```python
from build123d import *

# Parameters (mm, degrees)
ESBO_O1_R                  = 1.75
ESBO_O1_R_2                = 11.5
ESBO_O1_R_3                = 4
ESBO_O1_R_4                = 2.25
RESSALTO_EXTRUS_O1_DEPTH   = 30
ESBO_O2_W                  = 43
ESBO_O2_H                  = 43
ESBO_O2_W_2                = 5.1
ESBO_O2_H_2                = 3
CORTE_EXTRUS_O1_DEPTH      = 22
ESBO_O3_R                  = 4.5
CORTE_EXTRUS_O2_DEPTH      = 3
CORTE_EXTRUS_O3_DEPTH      = 68.950349521
CORTE_EXTRUS_O3_DEPTH_BACK = 3
ESBO_O4_R                  = 1.5


with BuildPart() as part:
    # Esboço1 → Ressalto-extrusão1 (new body)
    with BuildSketch(Plane.XY):
        with BuildLine():
            Line((-26, 26), (26, 26))
            Line((26, 26), (47.462602, 10.027939539))
            ThreePointArc((47.462602, 10.027939539), (52.5, 0), (47.462602, -10.027939539))
            Line((47.462602, -10.027939539), (26, -26))
            Line((26, -26), (-26, -26))
            Line((-26, -26), (-47.462602, -10.027939539))
            ThreePointArc((-47.462602, -10.027939539), (-52.5, 0), (-47.462602, 10.027939539))
            Line((-47.462602, 10.027939539), (-26, 26))
        make_face()
        with Locations((-15.5, 15.5)):
            Circle(ESBO_O1_R, mode=Mode.SUBTRACT)
        with Locations((15.5, 15.5)):
            Circle(ESBO_O1_R, mode=Mode.SUBTRACT)
        with Locations((15.5, -15.5)):
            Circle(ESBO_O1_R, mode=Mode.SUBTRACT)
        with Locations((-15.5, -15.5)):
            Circle(ESBO_O1_R, mode=Mode.SUBTRACT)
        Circle(ESBO_O1_R_2, mode=Mode.SUBTRACT)
        with Locations((-40, 0)):
            Circle(ESBO_O1_R_3, mode=Mode.SUBTRACT)
        with Locations((40, 0)):
            Circle(ESBO_O1_R_3, mode=Mode.SUBTRACT)
        with Locations((-32.5, 7.5)):
            Circle(ESBO_O1_R_4, mode=Mode.SUBTRACT)
        with Locations((-32.5, -7.5)):
            Circle(ESBO_O1_R_4, mode=Mode.SUBTRACT)
        with Locations(Location((32.5, -7.5, 0), (0, 0, 180))):
            Circle(ESBO_O1_R_4, mode=Mode.SUBTRACT)
        with Locations(Location((32.5, 7.5, 0), (0, 0, 180))):
            Circle(ESBO_O1_R_4, mode=Mode.SUBTRACT)
    extrude(amount=RESSALTO_EXTRUS_O1_DEPTH)

    # Esboço2 → Corte-extrusão1 (cut)
    with BuildSketch(Plane.XY.offset(30)):
        Rectangle(ESBO_O2_W, ESBO_O2_H)
        with Locations((-40, 6.5)):
            Rectangle(ESBO_O2_W_2, ESBO_O2_H_2)
        with Locations((40, 6.5)):
            Rectangle(ESBO_O2_W_2, ESBO_O2_H_2)
    extrude(amount=-CORTE_EXTRUS_O1_DEPTH, mode=Mode.SUBTRACT)

    # Esboço3 → Corte-extrusão2 (cut)
    with BuildSketch(Plane(origin=(0, 0, 0), x_dir=(-1, 0, 0), z_dir=(0, 0, -1))):
        with Locations((-15.5, 15.5)):
            Circle(ESBO_O3_R)
        with Locations((15.5, 15.5)):
            Circle(ESBO_O3_R)
        with Locations((-15.5, -15.5)):
            Circle(ESBO_O3_R)
        with Locations((15.5, -15.5)):
            Circle(ESBO_O3_R)
    extrude(amount=-CORTE_EXTRUS_O2_DEPTH, mode=Mode.SUBTRACT)

    # Esboço4 → Corte-extrusão3 (cut, two sides: drawn at the far end of the back side and taken through both)
    with BuildSketch(Plane(origin=(0, 5, 0), x_dir=(1, 0, 0), z_dir=(0, 1, 0)).offset(-CORTE_EXTRUS_O3_DEPTH_BACK)):
        with Locations(Location((-40, -19, 0), (0, 0, 180))):
            Circle(ESBO_O4_R)
        with Locations((40, -19)):
            Circle(ESBO_O4_R)
    extrude(amount=CORTE_EXTRUS_O3_DEPTH + CORTE_EXTRUS_O3_DEPTH_BACK, mode=Mode.SUBTRACT)


solid = part.part
```
Source: CAD feature listing. Evaluate the final solid. Frame: model axes, mm. A direction names the side the tool comes from. Coordinates: 2 decimals unless noted, no trailing zeros. Loops run counter-clockwise (first coordinate to the right, second up) from the corner with the lowest first, then second, coordinate; pieces in that order, holes last. Notation, with made-up numbers: M 21.5,-30 L 56.5,-30 A14 cw 56.5,-11 Z; hole C 39,34.25 d7. An arc over 180 degrees is marked long. Use a Markdown table: item, result. Add a question column.
Q1. Draft query along X for faces 5 (the flat face through (36.882, -17.902, 14.79)), 6 (the cylindrical face through (30.354, 6.824, 14.79)), 7 (the flat face through (-36.581, -18.126, 14.79)). Return one class per face: pulls with the +X half, pulls with the -X half, needs draft (parallel to the pull), parting line crosses it, or undercut.
Q2. Section query C-C, the plane x = 15.5. Return loops of the section in (y, z).
Q3. Section query A-A, the plane x = 0. Return loops of the section in (y, z).
Q4. Material intervals for L1, parallel to Y at x = -15.5, z = 1.65; L2, parallel to Y at x = 0, z = 5; L3, parallel to Y at x = -2, z = 17, sorted ascending.
Q5. Access query for faces 1 (the flat face through (-37.45, 6, 19)), 2 (the cylindrical face through (-41.43, 4.49, 19.45)), 3 (the flat face through (-17.4, -15.4, 3)), 4 (the cylindrical face through (-14.6, -14, 5.5)). Directions: +Z, -Z, +X, -X, +Y, -Y. A direction counts if a zero-diameter tool reaches every point of the face in a straight line with its end or side. Return the directions, or none.
Q6. First-contact query: pin 1 (2.5 mm diameter, centred on x = -40, y = 7, fed in from +Z); pin 2 (2.5 mm diameter, centred on y = 6.5, z = 16, fed in from +X); pin 3 (7 mm diameter, centred on x = -15.5, y = 15.5, fed in from -Z); pin 4 (5 mm diameter, centred on y = -18, z = 11.5, fed in from +X). Flat tips, straight axial feed; report the tip coordinate or a pass-through.
Q7. Section query B-B, the plane z = 11. State how many separate pieces and enclosed holes the cut face has, and give its area (3 significant figures).
Q8. Section query D-D, the plane y = -15.5. Return loops of the section in (x, z), and give its area (3 significant figures).
Result:
| question | item | result |
|---|---|---|
| 1 | face 5 | pulls with the +X half |
| 1 | face 6 | undercut |
| 1 | face 7 | pulls with the -X half |
| 2 | outline | M -26,0 L -20,0 L -20,3 L -17.25,3 L -17.25,8 L -21.5,8 L -21.5,30 L -26,30 Z; M -13.75,3 L -11,3 L -11,0 L 11,0 L 11,3 L 13.75,3 L 13.75,8 L -13.75,8 Z; M 17.25,3 L 20,3 L 20,0 L 26,0 L 26,30 L 21.5,30 L 21.5,8 L 17.25,8 Z |
| 3 | outline | M -26,0 L -11.5,0 L -11.5,8 L -21.5,8 L -21.5,30 L -26,30 Z; M 11.5,0 L 26,0 L 26,30 L 21.5,30 L 21.5,8 L 11.5,8 Z |
| 4 | L1 | y = -26 to -20, -11 to 11, 20 to 26 |
| 4 | L2 | y = -26 to -11.5, 11.5 to 26 |
| 4 | L3 | y = -26 to -21.5, 21.5 to 26 |
| 5 | face 1 | +Z |
| 5 | face 2 | +Y |
| 5 | face 3 | -Z |
| 5 | face 4 | +Z, -Z |
| 6 | pin 1 | stops at z = 30 |
| 6 | pin 2 | stops at x = 51.34 |
| 6 | pin 3 | stops at z = 3 |
| 6 | pin 4 | stops at x = 40.11 |
| 7 | separate pieces | 1 |
| 7 | enclosed holes | 9 |
| 7 | area | 2,350 mm2 |
| 8 | outline | M -40.11,0 L -20,0 L -20,3 L -17.25,3 L -17.25,8 L -21.5,8 L -21.5,30 L -40.11,30 Z; M -13.75,3 L -11,3 L -11,0 L 11,0 L 11,3 L 13.75,3 L 13.75,8 L -13.75,8 Z; M 17.25,3 L 20,3 L 20,0 L 40.11,0 L 40.11,30 L 21.5,30 L 21.5,8 L 17.25,8 Z |
| 8 | area | 1,370 mm2 |
